Read the model definition and answer for the solid it produces. Units are mm, in the model's axes. Face numbers are marked on the shaded views. Round coordinates to 2 decimals unless told otherwise and drop trailing zeros. Write each loop counter-clockwise with the first axis right and the second up, starting at its lowest first coordinate (ties: lowest second). Pieces come first, ordered by that corner, then holes.
Autodesk Inventor part; units mm, degrees
ref_plane "YZ Plane" through (0, 0, 0) normal (1, 0, 0) x (0, 1, 0)
ref_plane "XZ Plane" through (0, 0, 0) normal (0, 1, 0) x (-1, 0, 0)
ref_plane "XY Plane" through (0, 0, 0) normal (0, 0, 1) x (1, 0, 0)
sketch "Sketch1" plane through (0, 0, 0) normal (0, 0, 1) x (1, 0, 0)
  circle A0 centre (0, 0) radius 63.5
  dimension "d0" = 127
extrude "Extrusion1" add sketch "Sketch1" along normal blind 2.54
sketch "Sketch2" plane through (0, 0, 2.54) normal (0, 0, 1) x (1, 0, 0)
  circle A0 centre (0, 0) radius 63.5
  circle A1 centre (0, 0) radius 19.05
  dimension "d3" = 38.1
extrude "Extrusion2" add sketch "Sketch2" along normal blind 254 contours A1
sketch "Sketch3" plane through (0, 0, 256.54) normal (0, 0, 1) x (1, 0, 0)
  circle A0 centre (0, 0) radius 19.05
  circle A1 centre (0, 0) radius 63.5
  dimension "d6" = 127
extrude "Extrusion3" add sketch "Sketch3" along normal blind 2.54 contours A0 | A1
properties part number "A solid metal acylinder"
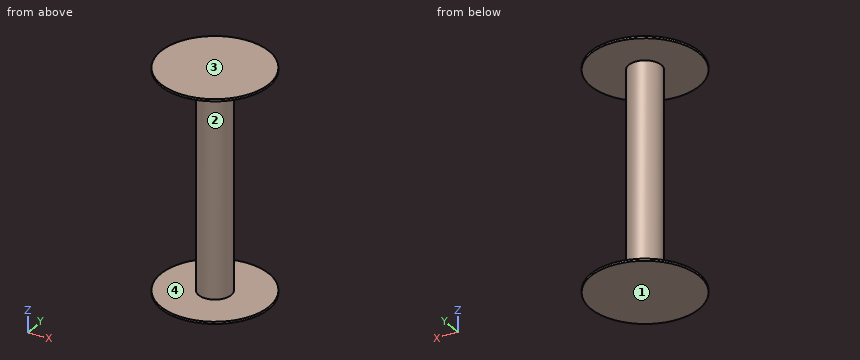
Q1. Straight lines are drawn through the part: probe 1 along Z at (x, y) = (-51.5, -14); probe 2 along Y at (x, z) = (12, 151); probe 3 along Y at (x, z) = (3, 185.5). For each, find the intervals that lie inside material, in ascending order.
Verdict:
probe 1: z = 0 to 2.54, 256.54 to 259.08
probe 2: y = -14.8 to 14.8
probe 3: y = -18.81 to 18.81
Q2. Flat-ended cylindrical pins translate along their axes: pin 1 Ø4 at (x, z) = (-7.5, 90.5) entering from +Y; pin 2 Ø10 at (x, z) = (6, 29.5) entering from -Y; pin 3 Ø1 at (y, z) = (4, 151.5) entering from -X. Find the tip coordinate at first contact, or state that the pin passes through.
Verdict:
pin 1: stops at y = 18.24
pin 2: stops at y = -19.02
pin 3: stops at x = -18.73
Q3. Determine the mould class of the marked faces 1, 2, 3 and 4 for opening direction Z: pulls with the +Z half, pulls with the -Z half, needs draft (parallel to the pull), parting line crosses it, or undercut.
Verdict:
face 1: pulls with the -Z half
face 2: undercut
face 3: pulls with the +Z half
face 4: undercut
Q4. Section C-C (x = -51) is taken. Determine the outline of the cut face in (y, z), then the cut area to 3 significant figures.
Verdict:
outline: (-37.83, 0) - (37.83, 0) - (37.83, 2.54) - (-37.83, 2.54) - close; (-37.83, 256.54) - (37.83, 256.54) - (37.83, 259.08) - (-37.83, 259.08) - close
area: 384 mm2
Q5. Section A-A (x = 0) is taken. Determine the outline of the cut face in (y, z), then the cut area to 3 significant figures.
Verdict:
outline: (-63.5, 0) - (63.5, 0) - (63.5, 2.54) - (19.05, 2.54) - (19.05, 256.54) - (63.5, 256.54) - (63.5, 259.08) - (-63.5, 259.08) - (-63.5, 256.54) - (-19.05, 256.54) - (-19.05, 2.54) - (-63.5, 2.54) - close
area: 10,300 mm2
Q6. Section B-B (y = -42) is taken. Determine the outline of the cut face in (x, z), then the cut area to 3 significant figures.
Verdict:
outline: (-47.63, 0) - (47.63, 0) - (47.63, 2.54) - (-47.63, 2.54) - close; (-47.63, 256.54) - (47.63, 256.54) - (47.63, 259.08) - (-47.63, 259.08) - close
area: 484 mm2
